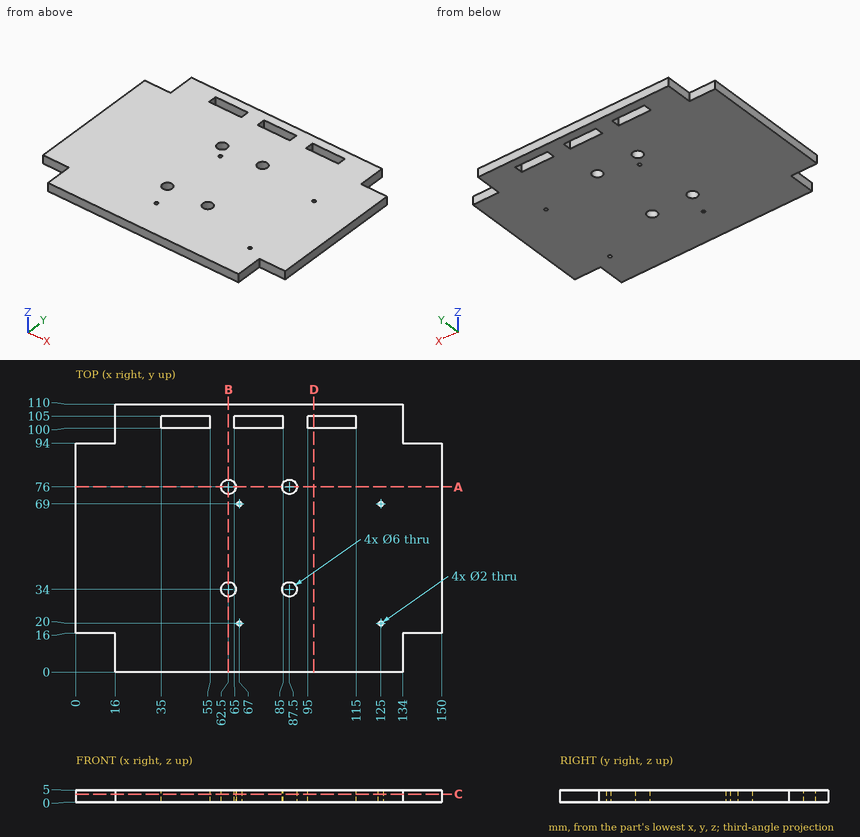
Source: three-view drawing plus pictorial views. Frame: mm from the lowest corner of the part. Coordinates: 2 decimals unless noted, no trailing zeros. Write each loop counter-clockwise with the first axis right and the second up, starting at its lowest first coordinate (ties: lowest second). Pieces come first, ordered by that corner, then holes. Notation, with made-up numbers: (-21, 78) - (16, 78) arc R17 cw to (16, 104) - close; hole circle Ø2 at (3, 34.5). An arc over 180 degrees is marked (long way). Return JSON: item names as keys, results as strings.
Item 1: Section query C-C (z = 3.4). Count the separate pieces of the cut face and the enclosed holes in it, and give its area (3 significant figures).
Completed:
{"separate pieces": "1", "enclosed holes": "11", "area": "15,100 mm2"}
Item 2: Section query B-B (x = 62.5). Output: boundary loops of the cut face in (y, z), and give its area (3 significant figures).
Completed:
{"outline": "(0, 0) - (31, 0) - (31, 5) - (0, 5) - close; (37, 0) - (73, 0) - (73, 5) - (37, 5) - close; (79, 0) - (110, 0) - (110, 5) - (79, 5) - close", "area": "490 mm2"}
Item 3: Section query D-D (x = 97.5). Output: boundary loops of the cut face in (y, z), and give its area (3 significant figures).
Completed:
{"outline": "(0, 0) - (100, 0) - (100, 5) - (0, 5) - close; (105, 0) - (110, 0) - (110, 5) - (105, 5) - close", "area": "525 mm2"}
Item 4: Section query A-A (y = 76). Output: boundary loops of the cut face in (x, z).
Completed:
{"outline": "(0, 0) - (59.5, 0) - (59.5, 5) - (0, 5) - close; (65.5, 0) - (84.5, 0) - (84.5, 5) - (65.5, 5) - close; (90.5, 0) - (150, 0) - (150, 5) - (90.5, 5) - close"}
Item 5: Pin query (flat end, axial travel): pin 1 Ø1.5 at (y, z) = (103.5, 2.5) entering from +X; pin 2 Ø2.5 at (y, z) = (10.5, 3.5) entering from -X; pin 3 Ø1.5 at (x, z) = (145, 2.5) entering from -Y. Return the tip coordinate at first contact, or that it passes through.
Completed:
{"pin 1": "stops at x = 134", "pin 2": "stops at x = 16", "pin 3": "stops at y = 16"}
Item 6: Line query: L1, parallel to Y at x = 62.5, z = 1.9; L2, parallel to Y at x = 125, z = 2.95; L3, parallel to X at y = 69, z = 3.4. Output: solid intervals per line, ascending.
Completed:
{"L1": "y = 0 to 31, 37 to 73, 79 to 110", "L2": "y = 0 to 19, 21 to 68, 70 to 110", "L3": "x = 0 to 66, 68 to 124, 126 to 150"}
